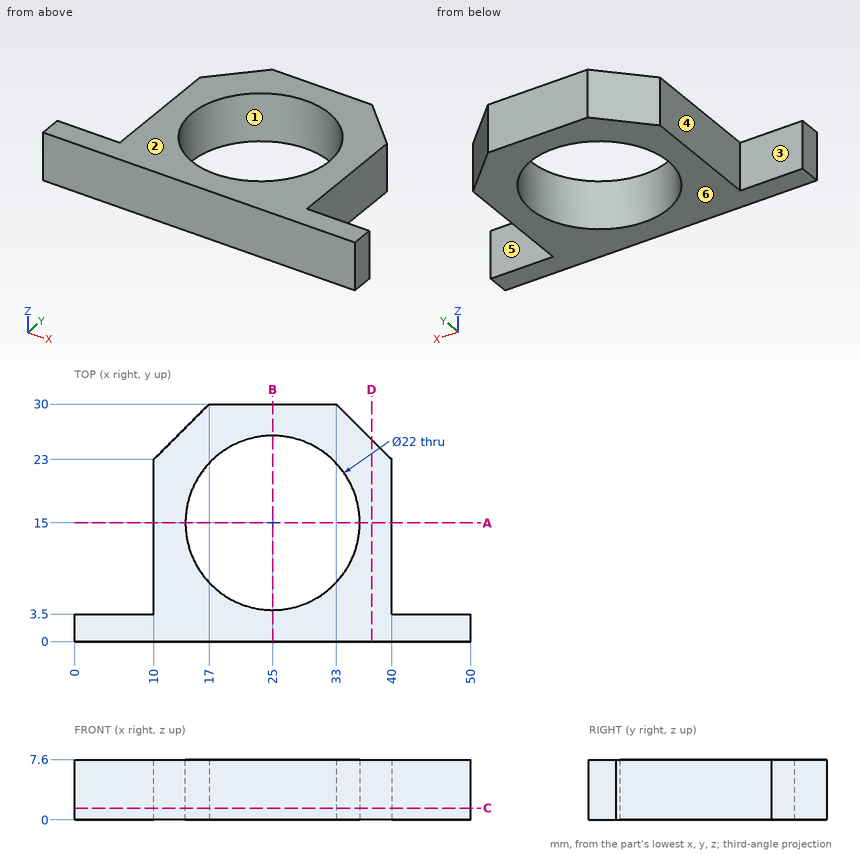
Design review of the part shown in the three views and the two pictorial views. Dimensions are in mm from the part's minimum x, y and z. A direction names the side the tool comes from. Give positions to 0.01 mm unless a question says otherwise; leave off trailing zeros. Loops run counter-clockwise (first coordinate to the right, second up) from the corner with the lowest first, then second, coordinate; pieces in that order, holes last. Notation, with made-up numbers: M -25.75,89 L -16.75,89 A8 cw -16.75,100 Z; hole C 74.25,48 d5. An arc over 180 degrees is marked long. Write item = value, one per line.
Q1. To check wall thickness, follow line 1 (Y direction, x = 25, z = 4.5); line 2 (X direction, y = 14, z = 6); line 3 (Y direction, x = 17, z = 1). State the ranges of each line that lie inside material, in increasing order. Write a range as [from, to].
Output values:
line_1 = [0, 4], [26, 30]
line_2 = [10, 14.05], [35.95, 40]
line_3 = [0, 7.45], [22.55, 30]
Q2. We need section B-B (x = 25). Give the boundary of the cut face in (y, z), plus the area to 3 significant figures.
Output values:
outline = M 0,0 L 4,0 L 4,7.6 L 0,7.6 Z; M 26,0 L 30,0 L 30,7.6 L 26,7.6 Z
area = 60.8 mm^2
Q3. We need section A-A (y = 15). Give the boundary of the cut face in (x, z), plus the area to 3 significant figures.
Output values:
outline = M 10,0 L 14,0 L 14,7.6 L 10,7.6 Z; M 36,0 L 40,0 L 40,7.6 L 36,7.6 Z
area = 60.8 mm^2
Q4. Insertion check: pin 1 (3 mm diameter, centred on y = 16, z = 5, fed in from +X); pin 2 (4 mm diameter, centred on y = 7, z = 6.5, fed in from -X); pin 3 (4 mm diameter, centred on y = 26, z = 1.5, fed in from +X). Each pin has a flat end and moves straight along its axis. Give the tip position at first contact, or say it passes through.
Output values:
pin_1 = 40
pin_2 = 10
pin_3 = 39
Q5. We need section D-D (x = 37.5). Give the boundary of the cut face in (y, z), plus the area to 3 significant figures.
Output values:
outline = M 0,0 L 25.5,0 L 25.5,7.6 L 0,7.6 Z
area = 194 mm^2
Q6. Draft analysis for pull direction Y (two halves, no side actions). For the marked faces 1, 2 and 3, state which applies: +Y half, -Y half, draft (parallel to the pull), parting line (faces both ways), or undercut.
Output values:
face_1 = undercut
face_2 = draft
face_3 = +Y half
Q7. For the marked faces 4, 5 and 6, list the 3-axis set-ups (+Z, -Z, +X, -X, +Y, -Y) from which the entire face can be reached by the end or side of a thin tool; tool diameter is ignored.
Output values:
face_4 = +Z, -Z, -X, +Y
face_5 = +Z, -Z, +X, +Y
face_6 = -Z, +X, -X, +Y, -Y
Q8. We need section C-C (z = 1.5). Give the boundary of the cut face in (x, y), plus the area to 3 significant figures.
Output values:
outline = M 0,0 L 50,0 L 50,3.5 L 40,3.5 L 40,23 L 33,30 L 17,30 L 10,23 L 10,3.5 L 0,3.5 Z; hole C 25,15 d22
area = 541 mm^2
